Could you check a few things on this model? Use its own coordinates, in mm. Face numbers are marked on the shaded views. A direction names the side the tool comes from. Give positions to 0.01 mm unless a question says otherwise; leave off trailing zeros. Write each loop counter-clockwise with the first axis right and the second up, starting at its lowest first coordinate (ties: lowest second). Pieces come first, ordered by that corner, then holes. Notation, with made-up numbers: M 25.25,0.25 L 78.25,0.25 A25 cw 78.25,21.25 Z; hole C 65,-14 d9. An arc over 180 degrees is marked long. Answer as CSV lines item,"result". Start each with the question number.
from build123d import *

# Parameters (mm, degrees)
IZIM1_W                     = 140
IZIM1_H                     = 40
Y_KSEKLIK_EKSTR_ZYON1_DEPTH = 60
IZIM2_W                     = 30
IZIM2_H                     = 60
KES_EKSTR_ZYON1_DEPTH       = 30
IZIM3_W                     = 60
IZIM3_H                     = 30
KES_EKSTR_ZYON2_DEPTH       = 61
KES_EKSTR_ZYON3_DEPTH       = 41
IZIM4_4_R                   = 20
Y_KSEKLIK_EKSTR_ZYON2_DEPTH = 5


with BuildPart() as part:
    # izim1 → Y_kseklik-Ekstr_zyon1 (new body)
    with BuildSketch(Plane.XY):
        with Locations((70, 20)):
            Rectangle(IZIM1_W, IZIM1_H)
    extrude(amount=Y_KSEKLIK_EKSTR_ZYON1_DEPTH)

    # izim2 → Kes-Ekstr_zyon1 (cut)
    with BuildSketch(Plane(origin=(0, 40, 0), x_dir=(1, 0, 0), z_dir=(0, 1, 0))):
        with Locations((15, -30)):
            Rectangle(IZIM2_W, IZIM2_H)
        with Locations((125, -30)):
            Rectangle(IZIM2_W, IZIM2_H)
    extrude(amount=-KES_EKSTR_ZYON1_DEPTH, mode=Mode.SUBTRACT)

    # izim3 → Kes-Ekstr_zyon2 (cut, through all)
    with BuildSketch(Plane.XY.offset(60)):
        with Locations((70, 15)):
            Rectangle(IZIM3_W, IZIM3_H)
    extrude(amount=-KES_EKSTR_ZYON2_DEPTH, mode=Mode.SUBTRACT)

    # izim4 → Kes-Ekstr_zyon3 (cut, through all)
    with BuildSketch(Plane(origin=(0, 40, 0), x_dir=(1, 0, 0), z_dir=(0, 1, 0))):
        with BuildLine():
            Line((56.339745962, -25), (61.339745962, -25))
            ThreePointArc((61.339745962, -25), (70, -20), (78.660254038, -25))
            Line((78.660254038, -25), (83.660254038, -25))
            Line((83.660254038, -25), (83.660254038, -35))
            Line((83.660254038, -35), (78.660254038, -35))
            ThreePointArc((78.660254038, -35), (70, -40), (61.339745962, -35))
            Line((61.339745962, -35), (56.339745962, -35))
            Line((56.339745962, -35), (56.339745962, -25))
        make_face()
    extrude(amount=-KES_EKSTR_ZYON3_DEPTH, mode=Mode.SUBTRACT)

    # izim4_4 → Y_kseklik-Ekstr_zyon2 (add)
    with BuildSketch(Plane(origin=(0, 40, 0), x_dir=(1, 0, 0), z_dir=(0, 1, 0))):
        with Locations((70, -30)):
            Circle(IZIM4_4_R)
        with BuildLine():
            Line((56.339745962, -25), (61.339745962, -25))
            ThreePointArc((61.339745962, -25), (70, -20), (78.660254038, -25))
            Line((78.660254038, -25), (83.660254038, -25))
            Line((83.660254038, -25), (83.660254038, -35))
            Line((83.660254038, -35), (78.660254038, -35))
            ThreePointArc((78.660254038, -35), (70, -40), (61.339745962, -35))
            Line((61.339745962, -35), (56.339745962, -35))
            Line((56.339745962, -35), (56.339745962, -25))
        make_face(mode=Mode.SUBTRACT)
    extrude(amount=Y_KSEKLIK_EKSTR_ZYON2_DEPTH)


solid = part.part
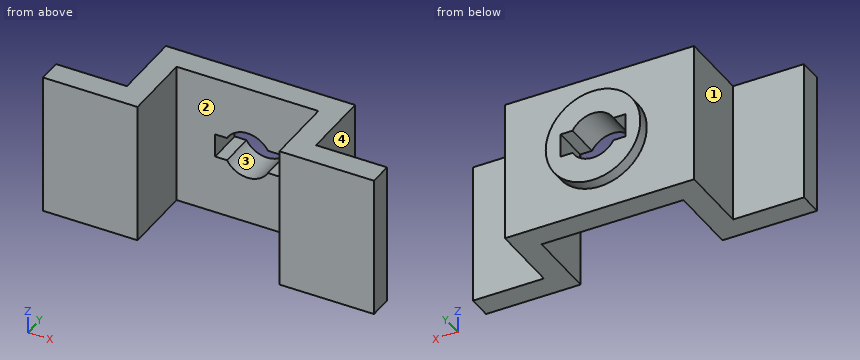
1. Will these pins go through, and if not, where does the flat tip stop? P1, Ø9, axis at y = 31, z = 43.5, coming from the +X side; P2, Ø6, axis at x = 99.5, z = 44.5, coming from the +Y side; P3, Ø15, axis at y = 21.5, z = 24.5, coming from the -X side.
2. Please list where these lines run through material, in increasing order: line 1 (X direction, y = 24, z = 5.5); line 2 (Z direction, x = 80, y = 31.5); line 3 (X direction, y = 6, z = 6).
3. On a 3-axis mill with a long thin cutter (end or side, diameter ignored), from which of +Z, -Z, +X, -X, +Y, -Y can I reach the whole of each face in a straight line? I mean the marked faces 1, 2, 3 and 4. Say none if no direction works.
4. Imagine slicing it at D-D, the plane y = 33. Please give me the cut outline in (x, z).
5. Imagine slicing it at B-B, the plane y = 12.5. Please give me the cut outline in (x, z), plus the area to 3 significant figures.
6. Imagine slicing it at C-C, the plane x = 70. Please give me the cut outline in (y, z), plus the area to 3 significant figures.
7. Imagine slicing it at A-A, the plane z = 30. Please give me the cut outline in (x, y), plus the area to 3 significant figures.
Solutions:
1,P1,"x = 110"
1,P2,"y = 40"
1,P3,"x = 30"
2,line 1,"30 to 40, 100 to 110"
2,line 2,"0 to 25, 35 to 60"
2,line 3,"0 to 40, 100 to 140"
3,face 1,"+Z, -Z, -X, +Y"
3,face 2,"+Z, -Z, -Y"
3,face 3,"+Y, -Y"
3,face 4,"+Z, -Z, +X, +Y"
4,outline,"M 30,0 L 110,0 L 110,60 L 30,60 Z; hole M 56.34,25 L 61.34,25 A10 ccw 78.66,25 L 83.66,25 L 83.66,35 L 78.66,35 A10 ccw 61.34,35 L 56.34,35 Z"
5,outline,"M 30,0 L 40,0 L 40,60 L 30,60 Z; M 100,0 L 110,0 L 110,60 L 100,60 Z"
5,area,"1,200 mm²"
6,outline,"M 30,0 L 40,0 L 40,10 L 45,10 L 45,20 L 30,20 Z; M 30,40 L 45,40 L 45,50 L 40,50 L 40,60 L 30,60 Z"
6,area,"500 mm²"
7,outline,"M 0,0 L 40,0 L 40,30 L 56.34,30 L 56.34,45 L 50,45 L 50,40 L 30,40 L 30,10 L 0,10 Z; M 83.66,30 L 100,30 L 100,0 L 140,0 L 140,10 L 110,10 L 110,40 L 90,40 L 90,45 L 83.66,45 Z"
7,area,"1,790 mm²"
